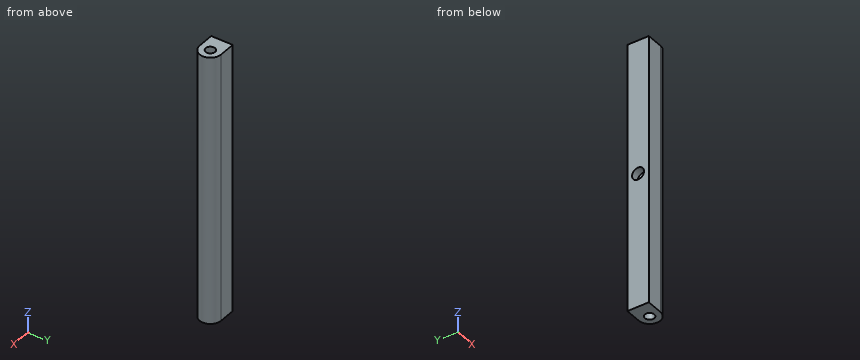
```python
from build123d import *

# Parameters (mm, degrees)
SKETCH1_R           = 17.5
BOSS_EXTRUDE1_DEPTH = 500
SKETCH2_R           = 22.5
CUT_EXTRUDE1_DEPTH  = 30


with BuildPart() as part:
    # Sketch1 → Boss-Extrude1 (new, symmetric)
    with BuildSketch(Plane.XY):
        with BuildLine():
            Line((0, 40), (-61.093968567, 40))
            Line((-61.093968567, 40), (-61.093968567, -40))
            Line((-61.093968567, -40), (0, -40))
            ThreePointArc((0, -40), (40, 0), (0, 40))
        make_face()
        Circle(SKETCH1_R, mode=Mode.SUBTRACT)
    extrude(amount=BOSS_EXTRUDE1_DEPTH, both=True)

    # Sketch2 → Cut-Extrude1 (cut)
    with BuildSketch(Plane.ZY.offset(61.093968567)):
        with Locations(Location((0, 0, 0), (0, 0, 270))):
            Circle(SKETCH2_R)
    extrude(amount=-CUT_EXTRUDE1_DEPTH, mode=Mode.SUBTRACT)


solid = part.part
```
For this review, take the finished solid that the model builds, in its own axes (mm). Coordinates: 2 decimals unless noted, no trailing zeros. Write each loop counter-clockwise with the first axis right and the second up, starting at its lowest first coordinate (ties: lowest second). Pieces come first, ordered by that corner, then holes.
(1) For pin 1 Ø1 at (x, z) = (11, 287) entering from +Y; pin 2 Ø5 at (x, z) = (3.5, 141.5) entering from -Y, all flat-tipped, find the tip position at first contact; note any pin that passes through.
(2) Add section B-B on z = 402.5. Give the boundary of the cut face in (x, y).
(3) Add section D-D on x = -41.5. Give the boundary of the cut face in (y, z).
(4) Wall thickness on probe 1 along X at (y, z) = (1, -432); probe 2 along Z at (x, y) = (-46.5, 6); probe 3 along Z at (x, y) = (-45.5, 0): over which ranges is each line inside the solid? List them lowest first.
(5) Add section C-C on x = 9. Give the boundary of the cut face in (y, z), then the cut area to 3 significant figures.
(6) Add section A-A on y = 0. Give the boundary of the cut face in (x, z).
Answer sheet:
1. pin 1: stops at y = 38.6
1. pin 2: stops at y = -39.99
2. outline: (-61.09, -40) - (0, -40) arc R40 ccw to (0, 40) - (-61.09, 40) - close; hole circle Ø35 at (0, 0)
3. outline: (-40, -500) - (40, -500) - (40, 500) - (-40, 500) - close; hole circle Ø45 at (0, 0)
4. probe 1: x = -61.09 to -17.47, 17.47 to 39.99
4. probe 2: z = -500 to -21.69, 21.69 to 500
4. probe 3: z = -500 to -22.5, 22.5 to 500
5. outline: (-38.97, -500) - (-15.01, -500) - (-15.01, 500) - (-38.97, 500) - close; (15.01, -500) - (38.97, -500) - (38.97, 500) - (15.01, 500) - close
5. area: 47,900 mm2
6. outline: (-61.09, -500) - (-17.5, -500) - (-17.5, 500) - (-61.09, 500) - (-61.09, 22.5) - (-31.09, 22.5) - (-31.09, -22.5) - (-61.09, -22.5) - close; (17.5, -500) - (40, -500) - (40, 500) - (17.5, 500) - close
